Can you work these out from the drawing? Everything is in mm from the part's minimum corner. A direction names the side the tool comes from. Give positions to 0.01 mm unless a question says otherwise; leave off trailing zeros. Loops run counter-clockwise (first coordinate to the right, second up) from the corner with the lowest first, then second, coordinate; pieces in that order, holes last.
Q1. I need wall thicknesses on line 1 (X direction, y = 3.5, z = 2.5); line 2 (Z direction, x = 10, y = 5.05); line 3 (X direction, y = 9.5, z = 6). Which ranges of each line are inside material? Lowest first, please.
Q2. If we section it at D-D (x = 25.5): Please give me the cut outline in (y, z).
Q3. We'd pull the mould along Z, two halves only. Please class the marked faces 6, 7 and 8: +Z half, -Z half, draft (parallel to the pull), parting line (faces both ways), or undercut.
Q4. For the marked faces 1, 2, 3, 4 and 5, which set-ups out of +Z, -Z, +X, -X, +Y, -Y let a thin tool reach every point of the face, with its end or its side?
Q5. If we section it at C-C (x = 21): Please give me the cut outline in (y, z).
Q6. If we section it at A-A (x = 10): Please give me the cut outline in (y, z), plus the area to 3 significant figures.
Q7. Will these pins go through, and if not, where does the flat tip stop? P1, Ø2, axis at x = 10.5, z = 9, coming from the +Y side; P2, Ø2.5, axis at x = 25.5, z = 5, coming from the +Y side; P3, Ø2, axis at y = 8, z = 5.5, coming from the -X side.
Q8. If we section it at B-B (x = 14.5): Please give me the cut outline in (y, z).
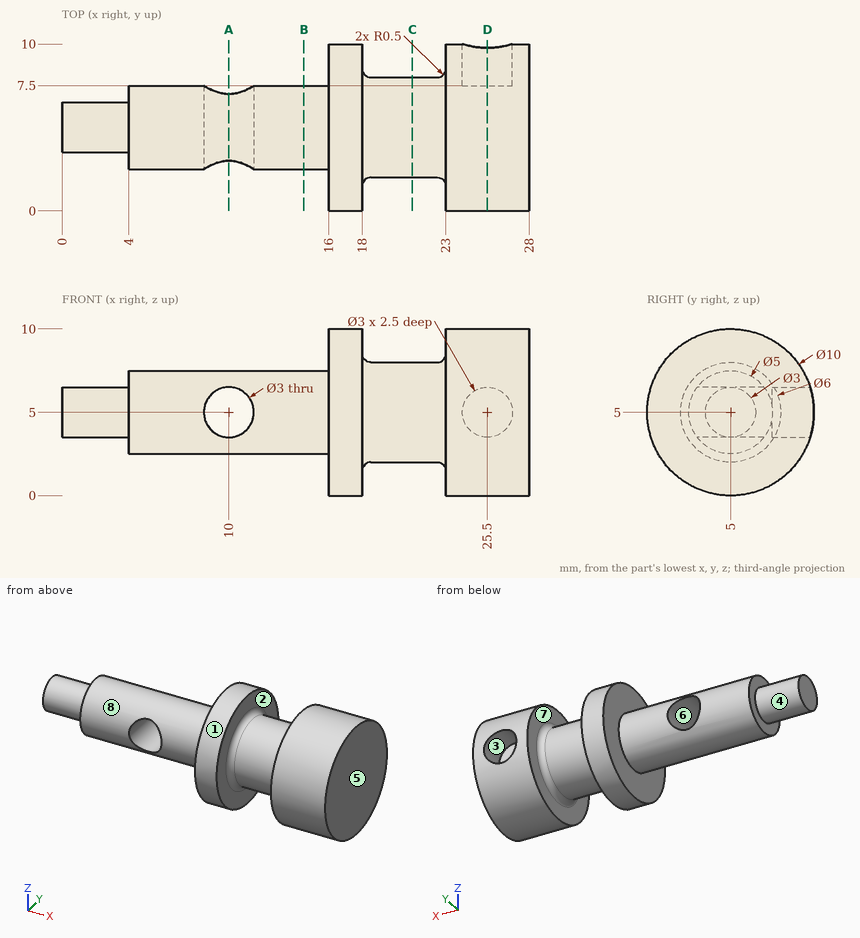
Check sheet entries:
1. line 1: x = 16 to 28
1. line 2: z = 2.5 to 3.5, 6.5 to 7.5
1. line 3: x = 16 to 18, 23 to 24.38, 26.62 to 28
2. outline: (7.5, 3.5) - (7.5, 6.5) - (9.77, 6.5) arc R5 ccw (long way) to (9.77, 3.5) - close
3. face 6: undercut
3. face 7: draft
3. face 8: parting line
4. face 1: +X, -X
4. face 2: none
4. face 3: +Y
4. face 4: -X
4. face 5: +Z, -Z, +X, +Y, -Y
5. outline: circle Ø6 at (5, 5)
6. outline: (3, 3.5) arc R2.5 ccw to (7, 3.5) - close; (3, 6.5) - (7, 6.5) arc R2.5 ccw to start
6. area: 5.59 mm2
7. P1: passes through
7. P2: stops at y = 7.5
7. P3: stops at x = 4
8. outline: circle Ø5 at (5, 5)
